Read the model definition and answer for the solid it produces. Units are mm, in the model's axes. A direction names the side the tool comes from. Give positions to 0.01 mm unless a question says otherwise; leave off trailing zeros. Write each question's results on one line, items separated by ' | '. Start each with the question number.
Item 1: Find the intervals of material crossed by line 1 (X direction, y = 92.5, z = 13.25); line 2 (Y direction, x = 29, z = 17.5), in increasing order.
Item 2: Which of the six approach directions +Z, -Z, +X, -X, +Y, -Y give full straight-line access (tool end or side, diameter ignored) to faces 4 (the flat face through (-4, -105, 10)), 5 (the flat face through (-50, 96, 10))?
Item 3: Determine the mould class of faces 1 (the flat face through (-1, 85, 10)), 2 (the flat face through (-325, 4, 10)), 3 (the flat face through (-189, 105, 10)) for opening direction X: +X half, -X half, draft (parallel to the pull), parting line (faces both ways), or undercut.
Item 4: Each of these flat-tipped pins is pushed along its axis until it touches: P1, Ø5, axis at x = -54.5, y = 20, coming from the -Z side; P2, Ø10, axis at x = 5.5, z = 11.5, coming from the +Y side. Where does it stop, or does it pass through?
```python
from build123d import *

# Parameters (mm, degrees)
F0_W     = 650
F0_H     = 210
F1_DEPTH = 20
F2_W     = 100
F2_H     = 20
F3_DEPTH = 20.001
F4_R     = 10
F5_R     = 2


with BuildPart() as f1:
    # F0 (on Top) → F1 (new body)
    with BuildSketch(Plane.XY):
        Rectangle(F0_W, F0_H)
    extrude(amount=F1_DEPTH)

    # F2 (on face) → F3 (cut, through all)
    with BuildSketch(Plane.XY.offset(20)):
        with Locations((0, 95)):
            Rectangle(F2_W, F2_H)
    extrude(amount=-F3_DEPTH, mode=Mode.SUBTRACT)

    # F4
    f4_edges = [f1.edges().sort_by_distance(p)[0] for p in [
        (-325, -105, 10),
        (325, -105, 10),
    ]]
    fillet(f4_edges, radius=F4_R)

    # F5
    f5_edges = [f1.edges().sort_by_distance(p)[0] for p in [
        (-50, 85, 10),
        (50, 85, 10),
    ]]
    fillet(f5_edges, radius=F5_R)


solid = f1.part
```
Findings:
1) line 1: -325 to -50, 50 to 325 | line 2: -105 to 85
2) face 4: +Z, -Z, +X, -X, -Y | face 5: +Z, -Z, +Y
3) face 1: undercut | face 2: -X half | face 3: draft
4) P1: z = 0 | P2: y = 85
